Check sheet for the modelled part. Datum: model origin and axes. Units: mm. Face numbers are marked on the shaded views. A direction names the side the tool comes from. Coordinates: 2 decimals unless noted, no trailing zeros. Loops run counter-clockwise (first coordinate to the right, second up) from the corner with the lowest first, then second, coordinate; pieces in that order, holes last. Notation, with made-up numbers: M -14,-19.75 L 13,-19.75 A3 ccw 13,-14.75 Z; hole C -4.5,-20.5 d1. An arc over 180 degrees is marked long. Write each question's results on one line, items separated by ' | '. Start each with the question number.
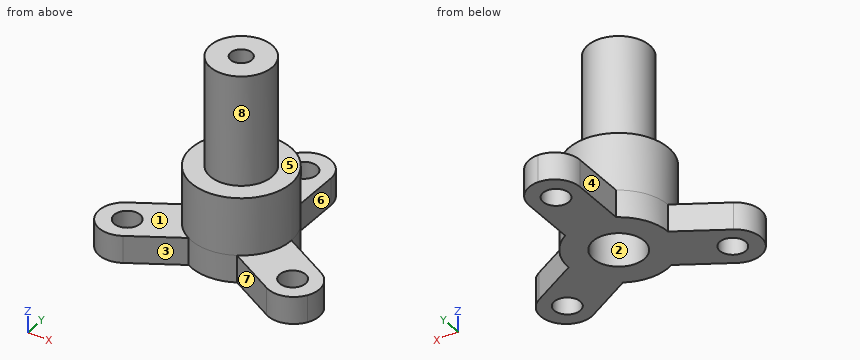
from build123d import *

# Parameters (mm, degrees)
F0_R     = 0.8255
F1_DEPTH = 1.7272
F2_R     = 3.175
F3_DEPTH = 3.6576
F4_R     = 1.9685
F5_DEPTH = 6.985
F6_R     = 0.6731
F7_DEPTH = 12.3708
F8_R     = 1.6256
F9_DEPTH = 4.572


with BuildPart() as f1:
    # F0 (on Top) → F1 (new body)
    with BuildSketch(Plane.XY):
        with BuildLine():
            ThreePointArc((-1.549093, -2.77145), (0, -3.175), (1.549093, -2.77145))
            Line((1.549093, -2.77145), (4.587475, -4.525661))
            ThreePointArc((4.587475, -4.525661), (5.821011, -4.688059), (6.808086, -3.93065))
            ThreePointArc((6.808086, -3.93065), (6.970484, -2.697114), (6.213075, -1.710039))
            Line((6.213075, -1.710039), (3.174693, 0.044171))
            ThreePointArc((3.174693, 0.044171), (2.749631, 1.5875), (1.6256, 2.727279))
            Line((1.6256, 2.727279), (1.6256, 6.2357))
            ThreePointArc((1.6256, 6.2357), (1.149473, 7.385173), (0, 7.8613))
            ThreePointArc((0, 7.8613), (-1.149473, 7.385173), (-1.6256, 6.2357))
            Line((-1.6256, 6.2357), (-1.6256, 2.727279))
            ThreePointArc((-1.6256, 2.727279), (-2.749631, 1.5875), (-3.174693, 0.044171))
            Line((-3.174693, 0.044171), (-6.213075, -1.710039))
            ThreePointArc((-6.213075, -1.710039), (-6.970484, -2.697114), (-6.808086, -3.93065))
            ThreePointArc((-6.808086, -3.93065), (-5.821011, -4.688059), (-4.587475, -4.525661))
            Line((-4.587475, -4.525661), (-1.549093, -2.77145))
        make_face()
        with Locations((-5.279291, -3.048)):
            Circle(F0_R, mode=Mode.SUBTRACT)
        with Locations((5.279291, -3.048)):
            Circle(F0_R, mode=Mode.SUBTRACT)
        with Locations((0, 6.096)):
            Circle(F0_R, mode=Mode.SUBTRACT)
    extrude(amount=F1_DEPTH)

    # F2 (on face) → F3 (join)
    with BuildSketch(Plane.XY.offset(1.7272)):
        Circle(F2_R)
    extrude(amount=F3_DEPTH)

    # F4 (on face) → F5 (join)
    with BuildSketch(Plane.XY.offset(5.3848)):
        Circle(F4_R)
    extrude(amount=F5_DEPTH)

    # F6 (on Top) → F7 (cut, through all)
    with BuildSketch(Plane.XY):
        Circle(F6_R)
    extrude(amount=F7_DEPTH, mode=Mode.SUBTRACT)

    # F8 (on face) → F9 (cut)
    with BuildSketch(Plane(origin=(0, 0, 0), x_dir=(1, 0, 0), z_dir=(0, 0, -1))):
        Circle(F8_R)
    extrude(amount=-F9_DEPTH, mode=Mode.SUBTRACT)


solid = f1.part
1) Section check A-A (x = -5). Enter the section's corners in (y, z).
2) Section check B-B (z = 3.25). Enter the section's corners in (x, y) (3 decimals), then the cut area to 3 significant figures.
3) Release check for a two-part mould opening along X. For the marked faces 6, 7 and 8 record: +X half, -X half, draft (parallel to the pull), parting line (faces both ways), or undercut.
4) Section check D-D (x = 5.5). Enter the section's corners in (y, z).
5) Thickness scan on probe 1 along Y at (x, z) = (0, 1.2) (1 decimal); probe 2 along Y at (x, z) = (0, 3.35) (3 decimals); probe 3 along Y at (x, z) = (0, 9.5). Record the ranges inside material, lowest first.
6) Section check C-C (y = 1.25). Enter the section's corners in (x, z), then the cut area to 3 significant figures.
7) Gauge pin test, flat ends, axial feed: P1, Ø2.5, axis at x = -0.5, y = 5, coming from the +Z side; P2, Ø1.4, axis at y = 5, z = 1, coming from the -X side; P3, Ø0.9, axis at y = 4, z = 0.5, coming from the +X side; P4, Ø0.8, axis at x = 0, y = 0, coming from the +Z side. Record the tip position at first contact, or that the pin passes through.
8) Set-up check for the marked faces 1, 2, 3, 4 and 5: record each of +Z, -Z, +X, -X, +Y, -Y from which the full face is reachable in a straight line by a thin tool's end or side.
Return value:
1) outline: M -4.69,0 L -3.82,0 L -3.82,1.73 L -4.69,1.73 Z; M -2.27,0 L -1.01,0 L -1.01,1.73 L -2.27,1.73 Z
2) outline: C 0,0 d6.35; hole C 0,0 d3.251 | area: 23.4 mm2
3) face 6: +X half | face 7: undercut | face 8: parting line
4) outline: M -4.74,0 L -3.84,0 L -3.84,1.73 L -4.74,1.73 Z; M -2.25,0 L -1.3,0 L -1.3,1.73 L -2.25,1.73 Z
5) probe 1: y = -3.2 to -1.6, 1.6 to 5.3, 6.9 to 7.9 | probe 2: y = -3.175 to -1.626, 1.626 to 3.175 | probe 3: y = -1.97 to -0.67, 0.67 to 1.97
6) outline: M -2.92,0 L -1.04,0 L -1.04,4.57 L 1.04,4.57 L 1.04,0 L 2.92,0 L 2.92,5.38 L 1.52,5.38 L 1.52,12.37 L -1.52,12.37 L -1.52,5.38 L -2.92,5.38 Z | area: 43.2 mm2
7) P1: stops at z = 1.73 | P2: stops at x = -1.63 | P3: stops at x = 1.63 | P4: passes through
8) face 1: +Z, -X, -Y | face 2: -Z | face 3: +Z, -Z, -Y | face 4: +Z, -Z, -X, +Y | face 5: +Z
